Print and shaded views of the part. All mm, measured from the part's lowest x, y and z. Round coordinates to 2 decimals unless told otherwise and drop trailing zeros. Loops run counter-clockwise (first coordinate to the right, second up) from the corner with the lowest first, then second, coordinate; pieces in that order, holes last. Notation, with made-up numbers: (8.5, 87) -> (26.5, 87) arc R33 ccw to (26.5, 121) -> close; hole circle Ø4 at (89, 11). An arc over 180 degrees is marked (long way). Answer as CSV lines item,"result".
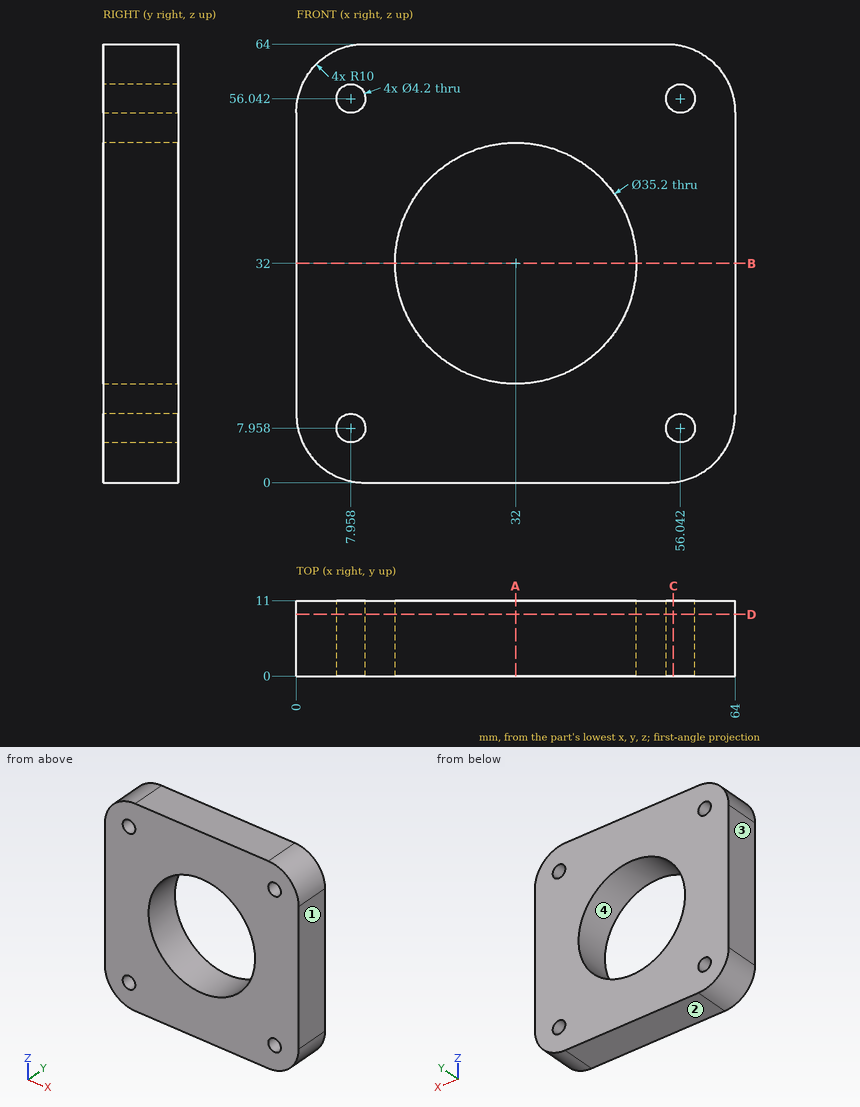
Q1. Two-plate mould, pull along X, no slides. Class the marked faces 1, 2, 3 and 4: pulls with the +X half, pulls with the -X half, needs draft (parallel to the pull), parting line crosses it, or undercut.
Results:
face 1,"pulls with the +X half"
face 2,"needs draft"
face 3,"pulls with the -X half"
face 4,"undercut"
Q2. Probe L1, parallel to X at y = 4.25, z = 32; L2, parallel to X at y = 7.25, z = 57; L3, parallel to Z at x = 23.5, y = 0.75. List the from-to ranges inside material, lowest first. Write a range as [from, to].
Results:
L1,"[0, 14.4], [49.6, 64]"
L2,"[0.46, 6.09], [9.83, 54.17], [57.91, 63.54]"
L3,"[0, 16.59], [47.41, 64]"
Q3. Slice it at C-C, the plane x = 55. Count the separate pieces of the cut face and the enclosed holes in it, and give its area (3 significant figures).
Results:
separate pieces,"3"
enclosed holes,"0"
area,"623 mm2"
Q4. Slice it at B-B, the plane z = 32. Give the cut face in (x, y), and give its area (3 significant figures).
Results:
outline,"(0, 0) -> (14.4, 0) -> (14.4, 11) -> (0, 11) -> close; (49.6, 0) -> (64, 0) -> (64, 11) -> (49.6, 11) -> close"
area,"317 mm2"
Q5. Slice it at D-D, the plane y = 9. Give the cut face in (x, z).
Results:
outline,"(0, 10) arc R10 ccw to (10, 0) -> (54, 0) arc R10 ccw to (64, 10) -> (64, 54) arc R10 ccw to (54, 64) -> (10, 64) arc R10 ccw to (0, 54) -> close; hole circle Ø4.2 at (7.96, 7.96); hole circle Ø4.2 at (7.96, 56.04); hole circle Ø35.2 at (32, 32); hole circle Ø4.2 at (56.04, 7.96); hole circle Ø4.2 at (56.04, 56.04)"
Q6. Slice it at A-A, the plane x = 32. Give the cut face in (y, z).
Results:
outline,"(0, 0) -> (11, 0) -> (11, 14.4) -> (0, 14.4) -> close; (0, 49.6) -> (11, 49.6) -> (11, 64) -> (0, 64) -> close"
